```python
from build123d import *

# Parameters (mm, degrees)
SALIENTE_EXTRUIR1_DEPTH = 3


with BuildPart() as part:
    # Croquis1 → Saliente-Extruir1 (new body)
    with BuildSketch(Plane.XY):
        with BuildLine():
            Line((0, 22.001027223), (-5, 22.001027223))
            Line((-5, 22.001027223), (-5, 12.001027223))
            ThreePointArc((-5, 12.001027223), (-4.121320344, 9.87970688), (-2, 9.001027223))
            Line((-2, 9.001027223), (12, 9.001027223))
            ThreePointArc((12, 9.001027223), (14.121320344, 9.87970688), (15, 12.001027223))
            Line((15, 12.001027223), (15, 22.001027223))
            Line((15, 22.001027223), (10, 22.001027223))
            Line((10, 22.001027223), (10, 19.001027223))
            Line((10, 19.001027223), (0, 19.001027223))
            Line((0, 19.001027223), (0, 22.001027223))
        make_face()
    extrude(amount=SALIENTE_EXTRUIR1_DEPTH)


solid = part.part
```
The listing builds one solid part. Answer for the finished solid, in the listing's coordinates (mm). A direction names the side the tool comes from. Round coordinates to 2 decimals unless told otherwise and drop trailing zeros. Order: outer loops, then holes, each group sorted by start corner. A loop starts at its lowest first (then second) coordinate and runs counter-clockwise, first axis right, second up. Notation, with made-up numbers: (83.5, 20.25) -> (98.5, 20.25) arc R18 ccw to (98.5, 51.25) -> close; hole circle Ø6 at (5, -26). An arc over 180 degrees is marked (long way). Answer as CSV lines item,"result".
Q1. A cutting plane is placed at B-B on x = 3.75. Determine the outline of the cut face in (y, z).
Computed values:
outline,"(9, 0) -> (19, 0) -> (19, 3) -> (9, 3) -> close"
Q2. Given pin 1 (3 mm diameter, centred on x = 0, y = 17.5, fed in from -Z), flat-ended and moving along its own axis, determine where the tip first touches the part or whether it passes through.
Computed values:
pin 1,"stops at z = 0"
Q3. A cutting plane is placed at C-C on y = 10.5. Determine the outline of the cut face in (x, z).
Computed values:
outline,"(-4.6, 0) -> (14.6, 0) -> (14.6, 3) -> (-4.6, 3) -> close"
Q4. Which of the six approach directions +Z, -Z, +X, -X, +Y, -Y give full straight-line access (tool end or side, diameter ignored) to faces 1 (the flat face through (5, 16, 3)), 2 (the flat face through (0, 20, 1))?
Computed values:
face 1,"+Z, +X, -X, +Y, -Y"
face 2,"+Z, -Z, +Y"
Q5. Consider line 1 (X direction, y = 20.5, z = 0.95); line 2 (Y direction, x = 7, z = 1.55); line 3 (Y direction, x = -2.5, z = 2.45). Determine where each line is inside the solid, lowest interval first. Write a range as from..to.
Computed values:
line 1,"x = -5..0, 10..15"
line 2,"y = 9..19"
line 3,"y = 9.04..22"
Q6. For a pull along X with two mould halves and no side action, classify faces 3 (the cylindrical face through (14.1, 9.86, 1.48)), 4 (the flat face through (5, 9.001, 1)), 5 (the flat face through (10, 21, 1)), 6 (the flat face through (5, 19.001, 1)) as +X half, -X half, draft (parallel to the pull), parting line (faces both ways), or undercut.
Computed values:
face 3,"+X half"
face 4,"draft"
face 5,"undercut"
face 6,"undercut"
Q7. A cutting plane is placed at A-A on z = 0.95. Determine the outline of the cut face in (x, y).
Computed values:
outline,"(-5, 12) arc R3 ccw to (-2, 9) -> (12, 9) arc R3 ccw to (15, 12) -> (15, 22) -> (10, 22) -> (10, 19) -> (0, 19) -> (0, 22) -> (-5, 22) -> close"
